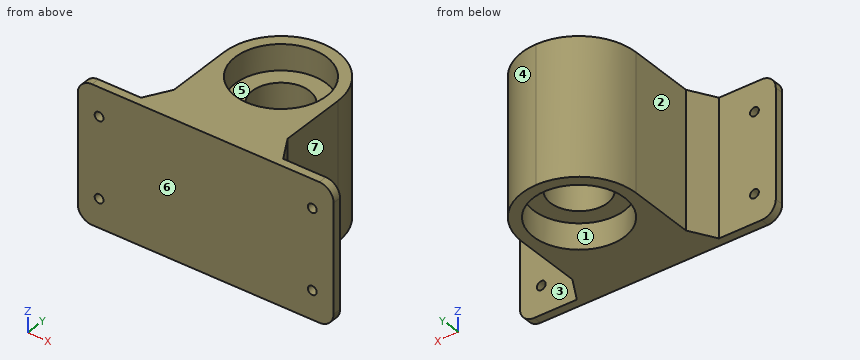
from build123d import *
from OCP.BRepFilletAPI import BRepFilletAPI_MakeChamfer

# Parameters (mm, degrees)
SKETCH_1_R          = 10
EXTRUDE_1_DEPTH     = 24
SKETCH_4_R          = 16.025
CUT_EXTRUDE_3_DEPTH = 9
SKETCH_5_W          = 48
SKETCH_5_H          = 3
EXTRUDE_2_DEPTH     = 25
CHAMFER_1_SIZE      = 5
CHAMFER_1_SIZE2     = 8.660254038
SKETCH_7_R          = 1.55
CUT_EXTRUDE_4_DEPTH = 76.00666637
FILLET_1_R          = 20
FILLET_2_R          = 5


with BuildPart() as part:
    # 草图1 → 凸台-拉伸1 (new, symmetric)
    with BuildSketch(Plane.XY):
        Polygon((-20, -35), (-20, 0), (-20, 20), (20, 20), (20, 0), (20, -35), align=None)
        Circle(SKETCH_1_R, mode=Mode.SUBTRACT)
    extrude(amount=EXTRUDE_1_DEPTH, both=True)

    # 草图4 → 切除-拉伸3 (cut)
    with BuildSketch(Plane(origin=(0, 0, -24), x_dir=(-1, 0, 0), z_dir=(0, 0, -1))):
        Circle(SKETCH_4_R)
    cut_extrude_3 = extrude(amount=-CUT_EXTRUDE_3_DEPTH, mode=Mode.SUBTRACT)

    # 镜向1: 切除-拉伸3 across plane
    add(cut_extrude_3.mirror(Plane.XY), mode=Mode.SUBTRACT)

    # 草图5 → 凸台-拉伸2 (add)
    with BuildSketch(Plane(origin=(20, 0, 0), x_dir=(0, 0, -1), z_dir=(1, 0, 0))):
        with Locations((0, -33.5)):
            Rectangle(SKETCH_5_W, SKETCH_5_H)
    extrude_2 = extrude(amount=EXTRUDE_2_DEPTH)

    # 镜向2: 凸台-拉伸2 across plane
    add(extrude_2.mirror(Plane.ZY))

    # 倒角1: one chamfer whose edges measure the first distance from different faces: ONE call of the kernel's chamfer builder (chamfer() names one face for all edges)
    chamfer_1_edges_1 = [part.edges().sort_by_distance(p)[0] for p in [
        (20, -32, 0),
    ]]
    chamfer_1_side_1 = [part.faces().sort_by_distance(p)[0] for p in [
        (32.5, -32, 0),
    ]]
    chamfer_1_edges_2 = [part.edges().sort_by_distance(p)[0] for p in [
        (-20, -32, 0),
    ]]
    chamfer_1_side_2 = [part.faces().sort_by_distance(p)[0] for p in [
        (-32.5, -32, 0),
    ]]
    chamfer_1 = BRepFilletAPI_MakeChamfer(part.part.solid().wrapped)
    for e in chamfer_1_edges_1:
        chamfer_1.Add(CHAMFER_1_SIZE, CHAMFER_1_SIZE2, e.wrapped, chamfer_1_side_1[0].wrapped)  # the first distance lies on this face
    for e in chamfer_1_edges_2:
        chamfer_1.Add(CHAMFER_1_SIZE, CHAMFER_1_SIZE2, e.wrapped, chamfer_1_side_2[0].wrapped)  # the first distance lies on this face
    add(Compound.cast(chamfer_1.Shape()), mode=Mode.REPLACE)

    # 草图7 → 切除-拉伸4 (cut, through all)
    with BuildSketch(Plane.XZ.offset(35)):
        with Locations(Location((37.5, 14, 0), (0, 0, 270))):
            Circle(SKETCH_7_R)
        with Locations(Location((37.5, -14, 0), (0, 0, 270))):
            Circle(SKETCH_7_R)
        with Locations(Location((-37.5, 14, 0), (0, 0, 90))):
            Circle(SKETCH_7_R)
        with Locations(Location((-37.5, -14, 0), (0, 0, 90))):
            Circle(SKETCH_7_R)
    extrude(amount=-CUT_EXTRUDE_4_DEPTH, mode=Mode.SUBTRACT)

    # 圆角1
    fillet_1_edges = [part.edges().sort_by_distance(p)[0] for p in [
        (20, 20, 0),
        (-20, 20, 0),
    ]]
    fillet(fillet_1_edges, radius=FILLET_1_R - 0.0001)  # a hair under: the kernel refuses the full size

    # 圆角2
    fillet_2_edges = [part.edges().sort_by_distance(p)[0] for p in [
        (45, -33.5, 24),
        (45, -33.5, -24),
        (-45, -33.5, 24),
        (-45, -33.5, -24),
    ]]
    fillet(fillet_2_edges, radius=FILLET_2_R)


solid = part.part
Can you work these out from the model? Positions are in its coordinate system, mm. Face numbers are marked on the shaded views. A direction names the side the tool comes from. Give positions to 0.01 mm unless a question says otherwise; leave off trailing zeros. Order: outer loops, then holes, each group sorted by start corner. A loop starts at its lowest first (then second) coordinate and runs counter-clockwise, first axis right, second up. Notation, with made-up numbers: M 80,-31.5 L 112,-31.5 A25 cw 112,-13.5 Z; hole C 19.5,60.25 d6. An arc over 180 degrees is marked long. Use a Markdown table: item, result. Add a question column.
Item 1: For the marked faces 1, 2 and 3, which set-ups out of +Z, -Z, +X, -X, +Y, -Y let a thin tool reach every point of the face, with its end or its side?
Item 2: If I drill on L1, parallel to Z at x = -37.5, y = -33.75; L2, parallel to X at y = -34, z = 14; L3, parallel to Y at x = 0, z = 21 (3 decimals), over which ranges is the centre line in solid material (lowest first)? Write a range as [from, to].
Item 3: Will these pins go through, and if not, where does the flat tip stop? pin 1 (4 mm diameter, centred on x = 37.5, z = -14, fed in from +Y); pin 2 (3 mm diameter, centred on x = 37.5, z = 14, fed in from +Y); pin 3 (22 mm diameter, centred on x = -34.5, z = -9.5, fed in from +Y); pin 4 (12 mm diameter, centred on y = -29, z = -17, fed in from -X).
Item 4: Suppose I cut it at B-B (x = -37.5). List the corners of the cut face in (y, z) for me, then the cut area to 3 significant figures.
Item 5: We'd pull the mould along Y, two halves only. Please class the marked faces 4, 5, 6 and 7: +Y half, -Y half, draft (parallel to the pull), parting line (faces both ways), or undercut.
Item 6: Suppose I cut it at A-A (z = -14). Count the separate pieces of the cut face and the enclosed holes in it, then the cut area to 3 significant figures.
Item 7: Suppose I cut it at D-D (x = 1.5). List the corners of the cut face in (y, z) for me.
Answer sheet:
| question | item | result |
|---|---|---|
| 1 | face 1 | -Z |
| 1 | face 2 | +Z, -Z, -X, +Y |
| 1 | face 3 | +Z, -Z, +X, +Y |
| 2 | L1 | z = [-24, -15.55], [-12.45, 12.45], [15.55, 24] |
| 2 | L2 | x = [-45, -39.05], [-35.95, 35.95], [39.05, 45] |
| 2 | L3 | y = [-35, -16.025], [16.025, 20] |
| 3 | pin 1 | stops at y = -32 |
| 3 | pin 2 | passes through |
| 3 | pin 3 | stops at y = -29.4 |
| 3 | pin 4 | stops at x = -45 |
| 4 | outline | M -35,-24 L -32,-24 L -32,-15.55 L -35,-15.55 Z; M -35,-12.45 L -32,-12.45 L -32,12.45 L -35,12.45 Z; M -35,15.55 L -32,15.55 L -32,24 L -35,24 Z |
| 4 | area | 125 mm² |
| 5 | face 4 | +Y half |
| 5 | face 5 | undercut |
| 5 | face 6 | -Y half |
| 5 | face 7 | draft |
| 6 | separate pieces | 3 |
| 6 | enclosed holes | 1 |
| 6 | area | 1,890 mm² |
| 7 | outline | M -35,-24 L -15.95,-24 L -15.95,-15 L -9.89,-15 L -9.89,15 L -15.95,15 L -15.95,24 L -35,24 Z; M 9.89,-15 L 15.95,-15 L 15.95,-24 L 19.94,-24 L 19.94,24 L 15.95,24 L 15.95,15 L 9.89,15 Z |
